```python
from build123d import *

# Parameters (mm, degrees)
EXTRUDE_1_DEPTH     = 4.4
CUT_EXTRUDE_1_DEPTH = 4.4
EXTRUDE_START       = -0.7
EXTRUDE_2_DEPTH     = 3
CUT_EXTRUDE_2_DEPTH = 3
SKETCH_7_W          = 6
SKETCH_7_H          = 6
EXTRUDE_4_DEPTH     = 1
FILLET_1_R          = 1
SKETCH_8_R          = 0.6
CUT_EXTRUDE_3_DEPTH = 1
CHAMFER_1_SIZE      = 0.1
SKETCH_9_R          = 1.1
CUT_EXTRUDE_4_DEPTH = 0.5


with BuildPart() as part:
    # Эскиз1 → Бобышка-Вытянуть1 (new body)
    with BuildSketch(Plane.XY):
        with BuildLine():
            Line((-40, 27), (40, 27))
            ThreePointArc((40, 27), (42.121320344, 26.121320344), (43, 24))
            Line((43, 24), (43, -24))
            ThreePointArc((43, -24), (42.121320344, -26.121320344), (40, -27))
            Line((40, -27), (-40, -27))
            ThreePointArc((-40, -27), (-42.121320344, -26.121320344), (-43, -24))
            Line((-43, -24), (-43, 24))
            ThreePointArc((-43, 24), (-42.121320344, 26.121320344), (-40, 27))
        make_face()
    extrude(amount=EXTRUDE_1_DEPTH)

    # Эскиз2 → Вырез-Вытянуть1 (cut)
    with BuildSketch(Plane.XY.offset(4.4)):
        with BuildLine():
            Line((-39.9, 26.5), (39.9, 26.5))
            ThreePointArc((39.9, 26.5), (41.738477631, 25.738477631), (42.5, 23.9))
            Line((42.5, 23.9), (42.5, -23.9))
            ThreePointArc((42.5, -23.9), (41.738477631, -25.738477631), (39.9, -26.5))
            Line((39.9, -26.5), (-39.9, -26.5))
            ThreePointArc((-39.9, -26.5), (-41.738477631, -25.738477631), (-42.5, -23.9))
            Line((-42.5, -23.9), (-42.5, 23.9))
            ThreePointArc((-42.5, 23.9), (-41.738477631, 25.738477631), (-39.9, 26.5))
        make_face()
    extrude(amount=-CUT_EXTRUDE_1_DEPTH, mode=Mode.SUBTRACT)

    # Эскиз4 → Бобышка-Вытянуть2 (add)
    with BuildSketch(Plane.XY.offset(4.4).offset(EXTRUDE_START)):
        with BuildLine():
            Line((-39.9, 26.5), (39.9, 26.5))
            ThreePointArc((39.9, 26.5), (41.738477631, 25.738477631), (42.5, 23.9))
            Line((42.5, 23.9), (42.5, -23.9))
            ThreePointArc((42.5, -23.9), (41.738477631, -25.738477631), (39.9, -26.5))
            Line((39.9, -26.5), (-39.9, -26.5))
            ThreePointArc((-39.9, -26.5), (-41.738477631, -25.738477631), (-42.5, -23.9))
            Line((-42.5, -23.9), (-42.5, 23.9))
            ThreePointArc((-42.5, 23.9), (-41.738477631, 25.738477631), (-39.9, 26.5))
        make_face()
    extrude(amount=-EXTRUDE_2_DEPTH)

    # Эскиз5 → Вырез-Вытянуть2 (cut)
    with BuildSketch(Plane.XY.offset(3.7)):
        with BuildLine():
            Line((-37, 23), (37, 23))
            ThreePointArc((37, 23), (38.414213562, 22.414213562), (39, 21))
            Line((39, 21), (39, -21))
            ThreePointArc((39, -21), (38.414213562, -22.414213562), (37, -23))
            Line((37, -23), (-37, -23))
            ThreePointArc((-37, -23), (-38.414213562, -22.414213562), (-39, -21))
            Line((-39, -21), (-39, 21))
            ThreePointArc((-39, 21), (-38.414213562, 22.414213562), (-37, 23))
        make_face()
    extrude(amount=-CUT_EXTRUDE_2_DEPTH, mode=Mode.SUBTRACT)

    # Эскиз7 → Бобышка-Вытянуть4 (add)
    with BuildSketch(Plane(origin=(0, 0, 0.7), x_dir=(-1, 0, 0), z_dir=(0, 0, -1))):
        with Locations((-36, 20)):
            Rectangle(SKETCH_7_W, SKETCH_7_H)
        with Locations((36, 20)):
            Rectangle(SKETCH_7_W, SKETCH_7_H)
        with Locations((36, -20)):
            Rectangle(SKETCH_7_W, SKETCH_7_H)
        with Locations((-36, -20)):
            Rectangle(SKETCH_7_W, SKETCH_7_H)
    extrude(amount=-EXTRUDE_4_DEPTH)

    # Скругление1
    fillet_1_edges = [part.edges().sort_by_distance(p)[0] for p in [
        (39, 17, 1.2),
        (33, 23, 1.2),
        (33, 17, 1.2),
        (-39, -17, 1.2),
        (-33, -23, 1.2),
        (-33, -17, 1.2),
        (-33, 23, 1.2),
        (-39, 17, 1.2),
        (-33, 17, 1.2),
        (33, -23, 1.2),
        (39, -17, 1.2),
        (33, -17, 1.2),
    ]]
    fillet(fillet_1_edges, radius=FILLET_1_R)

    # Эскиз8 → Вырез-Вытянуть3 (cut)
    with BuildSketch(Plane(origin=(0, 0, 0.7), x_dir=(-1, 0, 0), z_dir=(0, 0, -1))):
        with Locations((-36, 20)):
            Circle(SKETCH_8_R)
        with Locations((36, 20)):
            Circle(SKETCH_8_R)
        with Locations((36, -20)):
            Circle(SKETCH_8_R)
        with Locations((-36, -20)):
            Circle(SKETCH_8_R)
    extrude(amount=-CUT_EXTRUDE_3_DEPTH, mode=Mode.SUBTRACT)

    # Фаска1
    chamfer_1_edges = [part.edges().sort_by_distance(p)[0] for p in [
        (43, 0, 0),
        (42.121320344, -26.121320344, 0),
        (0, -27, 0),
        (-42.121320344, -26.121320344, 0),
        (42.121320344, -26.121320344, 4.4),
        (43, 0, 4.4),
        (42.121320344, 26.121320344, 4.4),
        (0, 27, 4.4),
        (-42.121320344, 26.121320344, 4.4),
        (-43, 0, 4.4),
        (-41.738477631, 25.738477631, 0),
        (0, 26.5, 0),
        (41.738477631, 25.738477631, 0),
        (42.5, 0, 0),
        (41.738477631, -25.738477631, 0),
        (0, -26.5, 0),
        (-41.738477631, -25.738477631, 0),
        (-42.5, 0, 0),
        (-41.738477631, 25.738477631, 4.4),
        (-42.5, 0, 4.4),
        (-41.738477631, -25.738477631, 4.4),
        (0, -26.5, 4.4),
        (41.738477631, -25.738477631, 4.4),
        (42.5, 0, 4.4),
        (41.738477631, 25.738477631, 4.4),
        (0, 26.5, 4.4),
        (-42.121320344, -26.121320344, 4.4),
        (-43, 0, 0),
        (0, -27, 4.4),
        (-42.121320344, 26.121320344, 0),
        (0, 27, 0),
        (42.121320344, 26.121320344, 0),
    ]]
    chamfer(chamfer_1_edges, length=CHAMFER_1_SIZE)

    # Эскиз9 → Вырез-Вытянуть4 (cut)
    with BuildSketch(Plane(origin=(0, 0, 0.7), x_dir=(-1, 0, 0), z_dir=(0, 0, -1))):
        with Locations((36, 20)):
            Circle(SKETCH_9_R)
        with Locations((36, -20)):
            Circle(SKETCH_9_R)
        with Locations((-36, -20)):
            Circle(SKETCH_9_R)
        with Locations((-36, 20)):
            Circle(SKETCH_9_R)
    extrude(amount=-CUT_EXTRUDE_4_DEPTH, mode=Mode.SUBTRACT)


solid = part.part
```
The listing builds one solid part. Answer for the finished solid, in the listing's coordinates (mm). A direction names the side the tool comes from. Round coordinates to 2 decimals unless told otherwise and drop trailing zeros. Loops run counter-clockwise (first coordinate to the right, second up) from the corner with the lowest first, then second, coordinate; pieces in that order, holes last. Notation, with made-up numbers: (25.5, -6) -> (79.5, -6) arc R8 cw to (79.5, 9) -> close; hole circle Ø5 at (-27.5, -30). An arc over 180 degrees is marked (long way). Use one line per item in the form item = value.
1. The part is cut by section A-A on y = 8. Determine the outline of the cut face in (x, z).
Answer key:
outline = (-43, 0.1) -> (-42.9, 0) -> (-42.6, 0) -> (-42.5, 0.1) -> (-42.5, 0.7) -> (-39, 0.7) -> (-39, 3.7) -> (-42.5, 3.7) -> (-42.5, 4.3) -> (-42.6, 4.4) -> (-42.9, 4.4) -> (-43, 4.3) -> close; (39, 0.7) -> (42.5, 0.7) -> (42.5, 0.1) -> (42.6, 0) -> (42.9, 0) -> (43, 0.1) -> (43, 4.3) -> (42.9, 4.4) -> (42.6, 4.4) -> (42.5, 4.3) -> (42.5, 3.7) -> (39, 3.7) -> close
2. Find the intervals of material crossed by probe 1 along Y at (x, z) = (36, 1.45); probe 2 along Y at (x, z) = (-36, 0.95); probe 3 along Y at (x, z) = (29, 3.75), in increasing order. Write a range as [from, to].
Answer key:
probe_1 = [-27, -20.6], [-19.4, -17], [17, 19.4], [20.6, 27]
probe_2 = [-27, -21.1], [-18.9, -17], [17, 18.9], [21.1, 27]
probe_3 = [-27, -26.5], [26.5, 27]
3. Flat-ended cylindrical pins translate along their axes: pin 1 Ø1.8 at (x, y) = (-36, -19.5) entering from -Z; pin 2 Ø1.3 at (x, y) = (-36, -20) entering from -Z; pin 3 Ø3.5 at (x, y) = (36.5, 19) entering from +Z. Find the tip coordinate at first contact, or state that the pin passes through.
Answer key:
pin_1 = 0.7
pin_2 = 1.2
pin_3 = 1.7
4. A tool of negligible diameter and unlimited length cuts with its end or side. For faces 5 (the cylindrical face through (-36.508, 19.024, 0.946)), 6 (the flat face through (39, 0, 2)), from which of +Z, -Z, +X, -X, +Y, -Y can it reach the whole face along a straight path? Write none if from no direction.
Answer key:
face_5 = -Z
face_6 = +Z
5. For a pull along X with two mould halves and no side action, classify faces 1 (the flat face through (35.28, -20.23, 1.2)), 2 (the cylindrical face through (41.759, -25.718, 0.404)), 3 (the flat face through (-1, 27, 2)), 4 (the flat face through (43, 0, 2)) as released by +X, released by -X, zero draft, split by the parting line, or undercut.
Answer key:
face_1 = undercut
face_2 = undercut
face_3 = zero draft
face_4 = released by +X
6. The part is cut by section B-B on x = 29. Determine the outline of the cut face in (y, z).
Answer key:
outline = (-27, 0.1) -> (-26.9, 0) -> (-26.6, 0) -> (-26.5, 0.1) -> (-26.5, 0.7) -> (-23, 0.7) -> (-23, 3.7) -> (-26.5, 3.7) -> (-26.5, 4.3) -> (-26.6, 4.4) -> (-26.9, 4.4) -> (-27, 4.3) -> close; (23, 0.7) -> (26.5, 0.7) -> (26.5, 0.1) -> (26.6, 0) -> (26.9, 0) -> (27, 0.1) -> (27, 4.3) -> (26.9, 4.4) -> (26.6, 4.4) -> (26.5, 4.3) -> (26.5, 3.7) -> (23, 3.7) -> close
